```python
from build123d import *

# Parameters (mm, degrees)
SKETCH1_R               = 75
BOSS_EXTRUDE1_DEPTH     = 60
BOSS_EXTRUDE2_DEPTH     = 20
SKETCH6_R               = 2.5
CUT_EXTRUDE4_DEPTH      = 145.896339998
CIRPATTERN1_COUNT       = 4
CUT_EXTRUDE3_DEPTH      = 145.896339998
CUT_EXTRUDE3_DEPTH_BACK = 145.896339998


with BuildPart() as part:
    # Sketch1 → Boss-Extrude1 (new body)
    with BuildSketch(Plane(origin=(0, 0, 0), x_dir=(0, 0, -1), z_dir=(1, 0, 0))):
        with Locations(Location((0, 0, 0), (0, 0, 180))):
            Circle(SKETCH1_R)
    extrude(amount=BOSS_EXTRUDE1_DEPTH)

    # Sketch5 → Boss-Extrude2 (add)
    with BuildSketch(Plane(origin=(0, 0, 0), x_dir=(0, 0, -1), z_dir=(1, 0, 0))):
        with BuildLine():
            Line((12.661492774, 95.827904611), (12.661492774, -93.388552108))
            ThreePointArc((12.661492774, -93.388552108), (0, -106.050044882), (-12.661492774, -93.388552108))
            Line((-12.661492774, -93.388552108), (-12.661492774, 95.827904611))
            ThreePointArc((-12.661492774, 95.827904611), (0, 108.489397385), (12.661492774, 95.827904611))
        make_face()
    extrude(amount=BOSS_EXTRUDE2_DEPTH)

    # Sketch6 → Cut-Extrude4 (cut, symmetric)
    with BuildSketch(Plane(origin=(0, 0, 0), x_dir=(0, 0, -1), z_dir=(1, 0, 0))):
        with Locations(Location((60.640992129, 0, 0), (0, 0, 180))):
            Circle(SKETCH6_R)
    cut_extrude4 = extrude(amount=CUT_EXTRUDE4_DEPTH, both=True, mode=Mode.SUBTRACT)

    # CirPattern1: Cut-Extrude4 ×4 about axis
    cirpattern1_axis = Axis((0, 0, 0.067453829), (1, 0, 0))
    for i in range(1, CIRPATTERN1_COUNT):
        add(cut_extrude4.rotate(cirpattern1_axis, i * 360 / CIRPATTERN1_COUNT), mode=Mode.SUBTRACT)

    # Sketch3 → Cut-Extrude3 (cut, two sides: drawn at the far end of the back side and taken through both)
    with BuildSketch(Plane.XY.offset(-CUT_EXTRUDE3_DEPTH_BACK)):
        with BuildLine():
            Line((0, 63.92351859), (0, -63.92351859))
            ThreePointArc((0, -63.92351859), (55, 0), (0, 63.92351859))
        make_face()
    extrude(amount=CUT_EXTRUDE3_DEPTH + CUT_EXTRUDE3_DEPTH_BACK, mode=Mode.SUBTRACT)


solid = part.part
```
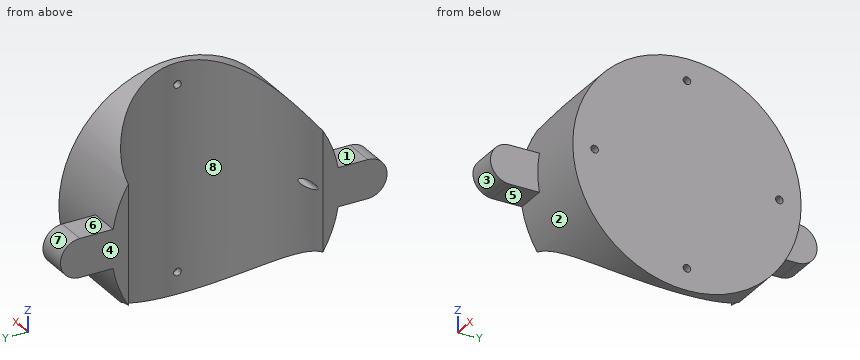
Geometry: final body of the model. Coordinates: model frame, mm. Face numbers are marked on the shaded views. A direction names the side the tool comes from. Round coordinates to 2 decimals unless told otherwise and drop trailing zeros. Order: outer loops, then holes, each group sorted by start corner. A loop starts at its lowest first (then second) coordinate and runs counter-clockwise, first axis right, second up. Notation, with made-up numbers: (-29, 23.5) -> (28, 23.5) arc R21 ccw to (28, 39.5) -> close; hole circle Ø1 at (73, 18.25). An arc over 180 degrees is marked (long way). Write each question's results on one line, items separated by ' | '.
Q1. Section query C-C (z = -24). Output: boundary loops of the cut face in (x, y), and give its area (3 significant figures).
Response values:
outline: (0, -71.06) -> (60, -71.06) -> (60, 71.06) -> (0, 71.06) -> (0, 63.92) arc R64.65 cw to (0, -63.92) -> close | area: 3,200 mm²
Q2. Pin query (flat end, axial travel): pin 1 Ø4 at (y, z) = (0, -60.64) entering from +X; pin 2 Ø21.5 at (x, y) = (12, -88) entering from -Z; pin 3 Ø4 at (x, z) = (17, 47) entering from -Y; pin 4 Ø5 at (x, y) = (52.5, -14) entering from -Z. Return the tip coordinate at first contact, or that it passes through.
Response values:
pin 1: through | pin 2: z = -12.66 | pin 3: y = -60 | pin 4: z = -74.05
Q3. Section query B-B (x = 44.5). Output: boundary loops of the cut face in (y, z), and give its area (3 significant figures).
Response values:
outline: (-35.32, -66.16) -> (-35.32, 66.16) arc R75 ccw to start; (35.32, -66.16) arc R75 ccw to (35.32, 66.16) -> close; hole circle Ø5 at (-60.71, 0.07); hole circle Ø5 at (60.71, 0.07) | area: 7,440 mm²
Q4. Section query D-D (y = 92). Output: boundary loops of the cut face in (x, z), and give its area (3 significant figures).
Response values:
outline: (0, -12.66) -> (20, -12.66) -> (20, 12.66) -> (0, 12.66) -> close | area: 506 mm²
Q5. Access query for the marked faces 1, 2, 3, 4 and 5. Directions: +Z, -Z, +X, -X, +Y, -Y. A direction counts if a zero-diameter tool reaches every point of the face in a straight line with its end or side. Return the directions, or none.
Response values:
face 1: +Z, +X, -X, -Y | face 2: +X | face 3: +X, -X, -Y | face 4: +Z, -Z, -X, +Y, -Y | face 5: -Z, +X, -X, -Y
Q6. Pull-direction query (Y, two-part tool) for the marked faces 6, 7 and 8; classes: released by +Y, released by -Y, zero draft, split by the parting line, or undercut.
Response values:
face 6: zero draft | face 7: released by +Y | face 8: undercut
Q7. Ray query, line 1 along Y through (x, z) = (19.5, 28); line 2 along Y through (x, z) = (43.5, 19); line 3 along X through (y, z) = (-3, -2). Return the intervals inside material, ascending.
Response values:
line 1: -69.58 to -57.7, 57.7 to 69.58 | line 2: -72.55 to -36.81, 36.81 to 72.55 | line 3: 54.93 to 60
Q8. Section query A-A (y = 0). Output: boundary loops of the cut face in (x, z).
Response values:
outline: (55, -75) -> (60, -75) -> (60, -63.14) -> (55, -63.14) -> close; (55, -58.14) -> (60, -58.14) -> (60, 58.28) -> (55, 58.28) -> close; (55, 63.28) -> (60, 63.28) -> (60, 75) -> (55, 75) -> close
